from build123d import *

# Parameters (mm, degrees)
SKETCH1_W           = 279.4
SKETCH1_H           = 76.2
BOSS_EXTRUDE1_DEPTH = 9.652
SKETCH2_R           = 3.175
SKETCH2_R_2         = 1.651
CUT_EXTRUDE1_DEPTH  = 9.652


with BuildPart() as part:
    # Sketch1 → Boss-Extrude1 (new body)
    with BuildSketch(Plane(origin=(0, 0, 0), x_dir=(1, 0, 0), z_dir=(0, 1, 0))):
        Rectangle(SKETCH1_W, SKETCH1_H)
    extrude(amount=BOSS_EXTRUDE1_DEPTH)

    # Sketch2 → Cut-Extrude1 (cut)
    with BuildSketch(Plane(origin=(0, 9.652, 0), x_dir=(1, 0, 0), z_dir=(0, 1, 0))):
        with Locations(Location((-127, 12.7, 0), (0, 0, 270))):
            Circle(SKETCH2_R)
        with Locations(Location((-44.45, 12.7, 0), (0, 0, 270))):
            Circle(SKETCH2_R_2)
        with Locations(Location((19.05, 12.7, 0), (0, 0, 270))):
            Circle(SKETCH2_R_2)
        with Locations(Location((127, 12.7, 0), (0, 0, 270))):
            Circle(SKETCH2_R)
        with Locations(Location((127, -12.7, 0), (0, 0, 90))):
            Circle(SKETCH2_R)
        with Locations(Location((19.05, -12.7, 0), (0, 0, 90))):
            Circle(SKETCH2_R_2)
        with Locations(Location((-44.45, -12.7, 0), (0, 0, 90))):
            Circle(SKETCH2_R_2)
        with Locations(Location((-127, -12.7, 0), (0, 0, 90))):
            Circle(SKETCH2_R)
    extrude(amount=-CUT_EXTRUDE1_DEPTH, mode=Mode.SUBTRACT)


solid = part.part
Source: CAD feature listing. Evaluate the final solid. Frame: model axes, mm. Coordinates: 2 decimals unless noted, no trailing zeros. Loops run counter-clockwise (first coordinate to the right, second up) from the corner with the lowest first, then second, coordinate; pieces in that order, holes last. Notation, with made-up numbers: M 10.25,-39 L 19.25,-39 A30 cw 19.25,-10 Z; hole C -39.75,69.5 d3. An arc over 180 degrees is marked long. Answer in a Markdown table with one row per item.
Q1. Section A-A on x = 127. Return the cut outline in (y, z) (3 decimals).
Answers below:
| item | result |
|---|---|
| outline | M 0,-38.1 L 9.652,-38.1 L 9.652,-15.875 L 0,-15.875 Z; M 0,-9.525 L 9.652,-9.525 L 9.652,9.525 L 0,9.525 Z; M 0,15.875 L 9.652,15.875 L 9.652,38.1 L 0,38.1 Z |
Q2. Ray query, probe 1 along X at (y, z) = (4.5, 12.7) (3 decimals); probe 2 along Z at (x, y) = (-126, 1.25); probe 3 along X at (y, z) = (5.75, 12). Return the intervals inside material, ascending. Write a range as from..to.
Answers below:
| item | result |
|---|---|
| probe 1 | x = -139.7..-130.175, -123.825..-46.101, -42.799..17.399, 20.701..123.825, 130.175..139.7 |
| probe 2 | z = -38.1..-15.71, -9.69..9.69, 15.71..38.1 |
| probe 3 | x = -139.7..-130.1, -123.9..-45.95, -42.95..17.55, 20.55..123.9, 130.1..139.7 |
Q3. Draft query along X for faces 1 (the flat face through (139.7, 5, 1)), 2 (the flat face through (-139.7, 5, 1)), 3 (the cylindrical face through (-130.15, 4.89, 13.11)), 4 (the flat face through (-2, 5, -38.1)). Return one class per face: pulls with the +X half, pulls with the -X half, needs draft (parallel to the pull), parting line crosses it, or undercut.
Answers below:
| item | result |
|---|---|
| face 1 | pulls with the +X half |
| face 2 | pulls with the -X half |
| face 3 | undercut |
| face 4 | needs draft |
Q4. First-contact query: pin 1 (2 mm diameter, centred on x = -44.45, z = -12.7, fed in from -Y). Flat tip, straight axial feed; report the tip coordinate or a pass-through.
Answers below:
| item | result |
|---|---|
| pin 1 | passes through |
